Input: dimensioned drawing with shaded views. Units: mm. Origin: part minimum x, y, z. Coordinates: 2 decimals unless noted, no trailing zeros. Order: outer loops, then holes, each group sorted by start corner. A loop starts at its lowest first (then second) coordinate and runs counter-clockwise, first axis right, second up.
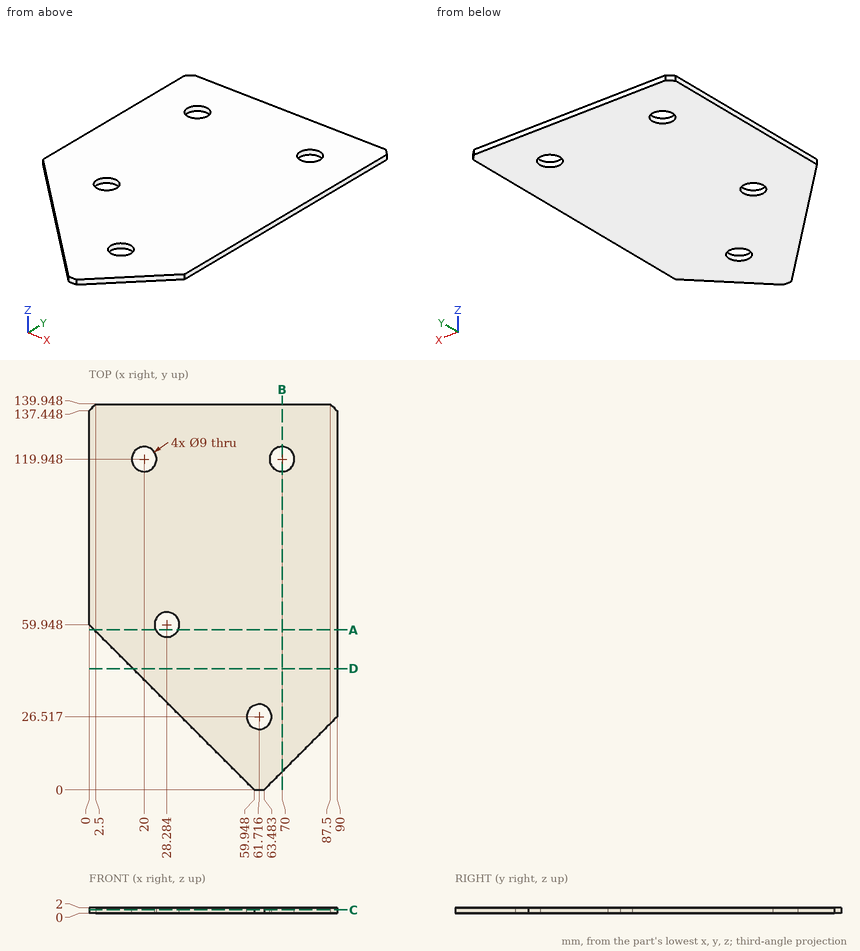
1. Section query B-B, the plane x = 70. Output: boundary loops of the cut face in (y, z).
2. Material intervals for line 1 along X through (y, z) = (116, 1.1) (1 decimal), sorted ascending.
3. Section query C-C, the plane z = 1.25. Output: boundary loops of the cut face in (x, y) (1 decimal).
4. Section query D-D, the plane y = 44. Output: boundary loops of the cut face in (x, z).
5. Contact query for flat-ended pins moving along their axis: P1, Ø8, axis at x = 20, y = 119.95, coming from the -Z side; P2, Ø12, axis at x = 9.5, y = 44, coming from the -Z side. Output: stop coordinate, or through.
6. Section query A-A, the plane y = 58. Output: boundary loops of the cut face in (x, z).
Answer key:
1. outline: (6.52, 0) - (115.45, 0) - (115.45, 2) - (6.52, 2) - close; (124.45, 0) - (139.95, 0) - (139.95, 2) - (124.45, 2) - close
2. line 1: x = 0 to 17.8, 22.2 to 67.8, 72.2 to 90
3. outline: (0, 59.9) - (59.9, 0) - (63.5, 0) - (90, 26.5) - (90, 137.4) - (87.5, 139.9) - (2.5, 139.9) - (0, 137.4) - close; hole circle Ø9 at (20, 119.9); hole circle Ø9 at (28.3, 59.9); hole circle Ø9 at (61.7, 26.5); hole circle Ø9 at (70, 119.9)
4. outline: (15.95, 0) - (90, 0) - (90, 2) - (15.95, 2) - close
5. P1: passes through
5. P2: stops at z = 0
6. outline: (1.95, 0) - (24.23, 0) - (24.23, 2) - (1.95, 2) - close; (32.34, 0) - (90, 0) - (90, 2) - (32.34, 2) - close
